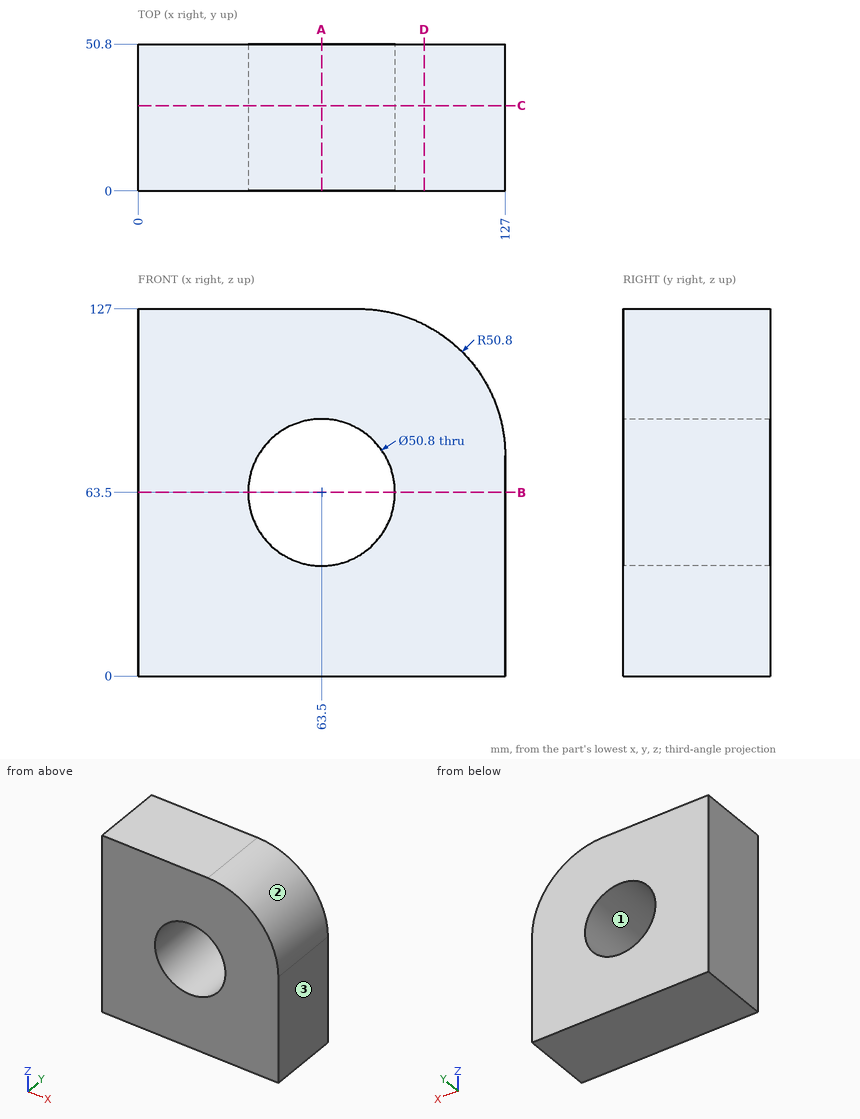
Part print with two shaded views. Sizes in mm from the minimum x, y, z corner. Round coordinates to 2 decimals unless told otherwise and drop trailing zeros. Loops run counter-clockwise (first coordinate to the right, second up) from the corner with the lowest first, then second, coordinate; pieces in that order, holes last. Notation, with made-up numbers: (-28, -37.5) - (8, -37.5) arc R32 ccw to (8, 1.5) - close; hole circle Ø8 at (71, 63.5). An arc over 180 degrees is marked (long way). Put each result on its own line as item: value.
1. Slice it at D-D on x = 99. List the corners of the cut face in (y, z).
Geometry check:
outline: (0, 0) - (50.8, 0) - (50.8, 121.6) - (0, 121.6) - close
2. Wall check: line 1 (X direction, y = 22, z = 63); line 2 (Z direction, x = 59.5, y = 13). Give the ranges that are in metal, low to high.
Geometry check:
line 1: 0 to 38.1, 88.9 to 127
line 2: 0 to 38.42, 88.58 to 127
3. Two-plate mould, pull along Z, no slides. Class the marked faces 1, 2 and 3: released by +Z, released by -Z, zero draft, split by the parting line, or undercut.
Geometry check:
face 1: undercut
face 2: released by +Z
face 3: zero draft
4. Pin check, flat tips, straight feed: P1, Ø2, axis at x = 102, y = 30, coming from the +Z side; P2, Ø1, axis at x = 114, y = 14.5, coming from the +Z side; P3, Ø12, axis at x = 85.5, y = 44, coming from the +Z side. Stop position of each tip, or through.
Geometry check:
P1: z = 120.54
P2: z = 110.69
P3: z = 126.89
5. Slice it at B-B on z = 63.5. List the corners of the cut face in (x, y), and give its area (3 significant figures).
Geometry check:
outline: (0, 0) - (38.1, 0) - (38.1, 50.8) - (0, 50.8) - close; (88.9, 0) - (127, 0) - (127, 50.8) - (88.9, 50.8) - close
area: 3,870 mm²
6. Slice it at C-C on y = 29.5. List the corners of the cut face in (x, z).
Geometry check:
outline: (0, 0) - (127, 0) - (127, 76.2) arc R50.8 ccw to (76.2, 127) - (0, 127) - close; hole circle Ø50.8 at (63.5, 63.5)
7. Slice it at A-A on x = 63.5. List the corners of the cut face in (y, z), and give its area (3 significant figures).
Geometry check:
outline: (0, 0) - (50.8, 0) - (50.8, 38.1) - (0, 38.1) - close; (0, 88.9) - (50.8, 88.9) - (50.8, 127) - (0, 127) - close
area: 3,870 mm²
